```python
from build123d import *

# Parameters (mm, degrees)
SKETCH1_W           = 25.4
SKETCH1_H           = 3.175
SKETCH1_R           = 3.175
SKETCH1_W_2         = 3.175
SKETCH1_H_2         = 32.279166667
SKETCH1_H_3         = 32.279166666
BOSS_EXTRUDE1_DEPTH = 3.175
SKETCH2_R           = 1.5
CUT_EXTRUDE1_DEPTH  = 394.059357795


with BuildPart() as part:
    # Sketch1 → Boss-Extrude1 (new body)
    # profile 1 of 13: a face of its own
    with BuildSketch(Plane.XY):
        Polygon((63.5, 387.35), (-63.5, 387.35), (-63.5, 355.070833333), (-63.5, 322.791666667), (-63.5, 290.5125), (-63.5, 258.233333333), (-63.5, 225.954166667), (-63.5, 193.675), (-63.5, 161.395833333), (-63.5, 129.116666667), (-63.5, 96.8375), (-63.5, 64.558333333), (-63.5, 32.279166667), (-63.5, 0), (63.5, 0), (63.5, 32.279166667), (63.5, 64.558333333), (63.5, 96.8375), (63.5, 129.116666667), (63.5, 161.395833333), (63.5, 193.675), (63.5, 225.954166667), (63.5, 258.233333333), (63.5, 290.5125), (63.5, 322.791666667), (63.5, 355.070833333), align=None)
        with Locations((0, 189.1665)):
            Rectangle(SKETCH1_W, SKETCH1_H, mode=Mode.SUBTRACT)
        with Locations((0, 203.454)):
            Circle(SKETCH1_R, mode=Mode.SUBTRACT)
    # profile 2 of 13: a face of its own
    with BuildSketch(Plane.XY):
        with Locations((-65.0875, 371.210416667)):
            Rectangle(SKETCH1_W_2, SKETCH1_H_2)
    # profile 3 of 13: a face of its own
    with BuildSketch(Plane.XY):
        with Locations((-65.0875, 306.652083334)):
            Rectangle(SKETCH1_W_2, SKETCH1_H_2)
    # profile 4 of 13: a face of its own
    with BuildSketch(Plane.XY):
        with Locations((-65.0875, 242.09375)):
            Rectangle(SKETCH1_W_2, SKETCH1_H_3)
    # profile 5 of 13: a face of its own
    with BuildSketch(Plane.XY):
        with Locations((-65.0875, 177.535416666)):
            Rectangle(SKETCH1_W_2, SKETCH1_H_2)
    # profile 6 of 13: a face of its own
    with BuildSketch(Plane.XY):
        with Locations((65.0875, 371.210416667)):
            Rectangle(SKETCH1_W_2, SKETCH1_H_2)
    # profile 7 of 13: a face of its own
    with BuildSketch(Plane.XY):
        with Locations((65.0875, 306.652083334)):
            Rectangle(SKETCH1_W_2, SKETCH1_H_2)
    # profile 8 of 13: a face of its own
    with BuildSketch(Plane.XY):
        with Locations((65.0875, 242.09375)):
            Rectangle(SKETCH1_W_2, SKETCH1_H_3)
    # profile 9 of 13: a face of its own
    with BuildSketch(Plane.XY):
        with Locations((65.0875, 177.535416666)):
            Rectangle(SKETCH1_W_2, SKETCH1_H_2)
    # profile 10 of 13: a face of its own
    with BuildSketch(Plane.XY):
        with Locations((65.0875, 112.977083334)):
            Rectangle(SKETCH1_W_2, SKETCH1_H_2)
    # profile 11 of 13: a face of its own
    with BuildSketch(Plane.XY):
        with Locations((-65.0875, 112.977083334)):
            Rectangle(SKETCH1_W_2, SKETCH1_H_2)
    # profile 12 of 13: a face of its own
    with BuildSketch(Plane.XY):
        with Locations((-65.0875, 48.41875)):
            Rectangle(SKETCH1_W_2, SKETCH1_H_3)
    # profile 13 of 13: a face of its own
    with BuildSketch(Plane.XY):
        with Locations((65.0875, 48.41875)):
            Rectangle(SKETCH1_W_2, SKETCH1_H_3)
    extrude(amount=BOSS_EXTRUDE1_DEPTH)

    # Sketch2 → Cut-Extrude1 (cut, through all)
    with BuildSketch(Plane.XY.offset(3.175)):
        with Locations((-44.45, 285.75)):
            Circle(SKETCH2_R)
        with Locations((44.45, 285.75)):
            Circle(SKETCH2_R)
        with Locations((-44.45, 15.875)):
            Circle(SKETCH2_R)
        with Locations((44.45, 15.875)):
            Circle(SKETCH2_R)
        with Locations((-44.45, 5.08)):
            Circle(SKETCH2_R)
        with Locations((44.45, 5.08)):
            Circle(SKETCH2_R)
    extrude(amount=-CUT_EXTRUDE1_DEPTH, mode=Mode.SUBTRACT)


solid = part.part
```
Check sheet for the modelled part. Datum: model origin and axes. Units: mm. Coordinates: 2 decimals unless noted, no trailing zeros. Loops run counter-clockwise (first coordinate to the right, second up) from the corner with the lowest first, then second, coordinate; pieces in that order, holes last. Notation, with made-up numbers: M -33,-20.75 L -17,-20.75 A32 cw -17,6.25 Z; hole C 35.25,60.25 d9. An arc over 180 degrees is marked long. Answer as a JSON object with one key per item and string values.
1. Depth check by flat-ended pin: P1, Ø1, axis at x = -65.5, z = 2, coming from the -Y side; P2, Ø8, axis at x = 48, y = 164, coming from the -Z side; P3, Ø1.6, axis at y = 142, z = 2, coming from the -X side; P4, Ø1.6, axis at y = 331, z = 1.5, coming from the +X side. Enter the tip coordinate at first touch or a pass-through.
Outcome:
{"P1": "y = 32.28", "P2": "z = 0", "P3": "x = -63.5", "P4": "x = 63.5"}
2. Scan lines: L1, parallel to Y at x = 44.45, z = 0.8 (3 decimals); L2, parallel to Y at x = -44, z = 0.3; L3, parallel to X at y = 285.75, z = 2.25. Record each from-to range of solid material in increasing order. Write a range as from..to.
Outcome:
{"L1": "0..3.58, 6.58..14.375, 17.375..284.25, 287.25..387.35", "L2": "0..3.65, 6.51..14.44, 17.31..284.32, 287.18..387.35", "L3": "-63.5..-45.95, -42.95..42.95, 45.95..63.5"}
3. Sectioned sample at A-A on z = 1.9. Count the separate pieces of the cut face and the enclosed holes in it, and give its area (3 significant figures).
Outcome:
{"separate pieces": "1", "enclosed holes": "8", "area": "50,300 mm²"}
4. Sectioned sample at B-B on y = 83.5. Record the cut outline in (x, z) (3 decimals).
Outcome:
{"outline": "M -63.5,0 L 63.5,0 L 63.5,3.175 L -63.5,3.175 Z"}
